from build123d import *

# Parameters (mm, degrees)
SKETCH1_R           = 2.075
SKETCH1_R_2         = 6.003208263
BOSS_EXTRUDE2_DEPTH = 8
FILLET1_R           = 2
BOSS_EXTRUDE3_START = -23
SKETCH2_R           = 16
SKETCH2_R_2         = 6.003208263
SKETCH2_R_3         = 2.001534735
SKETCH2_R_4         = 2.075
BOSS_EXTRUDE3_DEPTH = 23


with BuildPart() as part:
    # Sketch1 → Boss-Extrude2 (new body)
    with BuildSketch(Plane(origin=(0, 0, 0), x_dir=(1, 0, 0), z_dir=(0, 1, 0))):
        with BuildLine():
            Line((0, 44.83), (0, 36.83))
            ThreePointArc((0, 36.83), (36.83, 0), (0, -36.83))
            Line((0, -36.83), (0, -46.83))
            Line((0, -46.83), (0, -58.83))
            ThreePointArc((0, -58.83), (14.116701064, -87.229775601), (8, -56.110417137))
            Line((8, -56.110417137), (8, -44.110417137))
            ThreePointArc((8, -44.110417137), (44.649741882, 4.016148637), (0, 44.83))
        make_face()
        with Locations(Location((0.96696537, -64.081170969, 0), (0, 0, 270))):
            Circle(SKETCH1_R, mode=Mode.SUBTRACT)
        with Locations(Location((16.96696537, -64.081170969, 0), (0, 0, 270))):
            Circle(SKETCH1_R, mode=Mode.SUBTRACT)
        with Locations(Location((16.96696537, -80.081170969, 0), (0, 0, 270))):
            Circle(SKETCH1_R, mode=Mode.SUBTRACT)
        with Locations(Location((0.96696537, -80.081170969, 0), (0, 0, 270))):
            Circle(SKETCH1_R, mode=Mode.SUBTRACT)
        with Locations(Location((8.96696537, -72.081170969, 0), (0, 0, 270))):
            Circle(SKETCH1_R_2, mode=Mode.SUBTRACT)
    extrude(amount=BOSS_EXTRUDE2_DEPTH)

    # Fillet1
    fillet1_edges = [part.edges().sort_by_distance(p)[0] for p in [
        (0, 4, 58.83),
        (0, 4, 36.83),
        (0, 4, -36.83),
        (0, 4, -44.83),
        (8, 4, 44.110417137),
        (8, 4, 56.110417137),
    ]]
    fillet(fillet1_edges, radius=FILLET1_R)

    # Sketch2 → Boss-Extrude3 (add)
    with BuildSketch(Plane(origin=(0, 8, 0), x_dir=(1, 0, 0), z_dir=(0, 1, 0)).offset(BOSS_EXTRUDE3_START)):
        with Locations(Location((8.96696537, -72.081170969, 0), (0, 0, 86.709940875))):
            Circle(SKETCH2_R)
        with Locations(Location((8.96696537, -72.081170969, 0), (0, 0, 270))):
            Circle(SKETCH2_R_2, mode=Mode.SUBTRACT)
        with Locations(Location((16.96696537, -80.081170969, 0), (0, 0, 270))):
            Circle(SKETCH2_R_3, mode=Mode.SUBTRACT)
        with Locations(Location((16.96696537, -64.081170969, 0), (0, 0, 270))):
            Circle(SKETCH2_R_4, mode=Mode.SUBTRACT)
        with Locations(Location((0.96696537, -64.081170969, 0), (0, 0, 270))):
            Circle(SKETCH2_R_4, mode=Mode.SUBTRACT)
        with Locations(Location((0.96696537, -80.081170969, 0), (0, 0, 270))):
            Circle(SKETCH2_R_4, mode=Mode.SUBTRACT)
    extrude(amount=BOSS_EXTRUDE3_DEPTH)


solid = part.part
Can you work these out from the model? Positions are in its coordinate system, mm. A direction names the side the tool comes from. Coordinates: 2 decimals unless noted, no trailing zeros. Loops run counter-clockwise (first coordinate to the right, second up) from the corner with the lowest first, then second, coordinate; pieces in that order, holes last. Notation, with made-up numbers: M -32.75,12 L -15.75,12 A24 cw -15.75,26 Z; hole C -25.75,88.5 d4. An arc over 180 degrees is marked long. Return JSON: item names as keys, results as strings. Group by question number.
Item 1: If I drill on L1, parallel to Z at x = 9, y = -6.5; L2, parallel to Z at x = 13, y = 1.75; L3, parallel to Z at x = 11.5, y = 5, over which ranges is the centre line in solid material (lowest first)? Write a range as from..to.
Item 2: Imagine slicing it at C-C (z = 0). Please give me the cut outline in (x, y).
Item 3: Imagine slicing it at B-B (y = 3.75). Please give me the cut outline in (x, z) (3 decimals).
Item 4: Imagine slicing it at A-A (x = 6.5). Please give me the cut outline in (y, z).
Item 5: Imagine slicing it at D-D (x = 41.5). Please give me the cut outline in (y, z), and give its area (3 significant figures).
Item 6: I'm going to push flat-ended pins straight in: pin 1 Ø5 at (x, y) = (8.5, -4.5) entering from -Z; pin 2 Ø4 at (y, z) = (3.5, 47.5) entering from -X; pin 3 Ø4 at (x, z) = (14.5, 35) entering from -Y; pin 4 Ø4.5 at (x, z) = (16.97, 80.08) entering from -Y. Where does each tip first touch, or does it pass through?
Item 7: On a 3-axis mill with a long thin cutter (end or side, diameter ignored), from which of +Z, -Z, +X, -X, +Y, -Y can I reach the whole of each face in a straight line? I mean faces 1 (the cylindrical face through (15.75, -3.66, 78.49)), 2 (the flat face through (0, 4, 48)). Say none if no direction works.
Item 8: Thinking about a two-plate mould opening in X: for faces 3 (the cylindrical face through (17.958, -3.661, 85.316)), 4 (the cylindrical face through (10.77, -3.661, 77.807)), 5 (the flat face through (8, 4, 50)), which applies, released by +X, released by -X, zero draft, split by the parting line, or undercut?
Verdict:
{
 "1": {"L1": "z = 56.08..66.08, 78.08..88.08", "L2": "z = -42.9..-34.46, 34.46..42.9, 56.6..67.63, 76.53..87.56", "L3": "z = -43.33..-34.99, 34.99..43.33, 56.28..66.64, 77.52..87.88"},
 "2": {"outline": "M 36.83,0 L 44.83,0 L 44.83,8 L 36.83,8 Z"},
 "3": {"outline": "M -0.781,59.394 A2 cw 0,57.808 L 0,38.778 A2 ccw 1.897,36.781 A36.83 cw 1.897,-36.781 A2 ccw 0,-38.778 L 0,-42.783 A2 ccw 2.093,-44.781 A44.83 ccw 9.573,43.796 A2 cw 8,45.75 L 8,54.111 A2 cw 9.885,56.108 A16 ccw long Z; hole C 0.967,64.081 d4.15; hole C 0.967,80.081 d4.15; hole C 8.967,72.081 d12.006; hole C 16.967,64.081 d4.15; hole C 16.967,80.081 d4.003"},
 "4": {"outline": "M -15,56.27 L 0,56.27 L 0,36.25 L 8,36.25 L 8,66.61 L -15,66.61 Z; M -15,77.55 L 8,77.55 L 8,87.89 L -15,87.89 Z; M 0,-44.36 L 8,-44.36 L 8,-36.25 L 0,-36.25 Z"},
 "5": {"outline": "M 0,-16.96 L 8,-16.96 L 8,16.96 L 0,16.96 Z", "area": "271 mm^2"},
 "6": {"pin 1": "stops at z = 56.08", "pin 2": "stops at x = 0", "pin 3": "stops at y = 0", "pin 4": "stops at y = -15"},
 "7": {"face 1": "+Y, -Y", "face 2": "-Z, -X, +Y, -Y"},
 "8": {"face 3": "split by the parting line", "face 4": "undercut", "face 5": "released by +X"}
}
